CAD build for the part. Positions are in the model's coordinates, mm. A direction names the side the tool comes from. Coordinates: 2 decimals unless noted, no trailing zeros. Write each loop counter-clockwise with the first axis right and the second up, starting at its lowest first coordinate (ties: lowest second). Pieces come first, ordered by that corner, then holes. Notation, with made-up numbers: M 24,-23.5 L 37,-23.5 A35 cw 37,9.5 Z; hole C -40,-18.75 d1. An arc over 180 degrees is marked long. Answer as CSV lines item,"result". Start each with the question number.
```python
from build123d import *

# Parameters (mm, degrees)
F0_W          = 40.64
F0_H          = 40.64
F1_DEPTH      = 23.876
F2_SIZE2      = 10.16
F2_SIZE       = 16.51
F4_DEPTH      = 5.5372
F4_DEPTH_BACK = 35.052
F6_DEPTH      = 0.508
F7_T4_DEPTH   = 41.0469310155
F7_S5_R       = 17.3367265746
F7_T6_DEPTH   = 25
F7_T10_DEPTH  = 41.0469310155
F7_S11_R      = 17.3367265746
F7_T12_DEPTH  = 25
F7_T16_DEPTH  = 41.0469310155
F7_S17_R      = 17.3367265746
F7_T18_DEPTH  = 25
F7_T23_DEPTH  = 41.0469310155
F7_S24_R      = 17.3367265746
F7_T25_DEPTH  = 25
F7_T30_DEPTH  = 41.0469310155
F7_S31_R      = 17.3367265746
F7_T32_DEPTH  = 25
F7_T37_DEPTH  = 41.0469310155
F7_S39_R      = 17.3367265746
F7_T40_DEPTH  = 25
F7_T44_DEPTH  = 41.0469310155
F7_S46_R      = 17.3367265746
F7_T47_DEPTH  = 25
F7_T51_DEPTH  = 41.0469310155
F7_S53_R      = 17.3367265746
F7_T54_DEPTH  = 25


# Not quite as in the source:
# - a fillet or chamfer that OpenCascade refuses, or shapes differently, is made with other operations: its cross-section is extruded or revolved along the edge and cut away or added


with BuildPart() as f1:
    # F0 (on Top) → F1 (new body)
    with BuildSketch(Plane.XY):
        with Locations((-20.32, 14.8309261845)):
            Rectangle(F0_W, F0_H)
    extrude(amount=F1_DEPTH)

    # F2
    f2_edges = [f1.edges().sort_by_distance(p)[0] for p in [
        (0, 14.830926, 23.876),
        (-20.32, 35.150926, 23.876),
        (-40.64, 14.830926, 23.876),
        (-20.32, -5.489074, 23.876),
    ]]
    chamfer(f2_edges, length=F2_SIZE, length2=F2_SIZE2)

    # F3 (on Front) → F4 (join, two sides)
    with BuildSketch(Plane.XZ) as f4_sk:
        with BuildLine():
            Line((-19.622727835, 21.5899987397), (-21.017272165, 21.5899987397))
            ThreePointArc((-21.017272165, 21.5899987397), (-32.4394065874, 17.2953936781), (-38.2026230943, 6.5392734254))
            Line((-38.2026230943, 6.5392734254), (-2.4373769057, 6.5392734254))
            ThreePointArc((-2.4373769057, 6.5392734254), (-8.2005934126, 17.2953936781), (-19.622727835, 21.5899987397))
        make_face()
    extrude(amount=F4_DEPTH)
    extrude(f4_sk.sketch, amount=-F4_DEPTH_BACK)

    # F5 (on face) → F6 (cut)
    with BuildSketch(Plane.XY.offset(23.876)):
        with BuildLine():
            Line((-20.32, 11.3146617191), (-20.32, 20.958676386))
            Line((-20.32, 20.958676386), (-22.098, 20.958676386))
            ThreePointArc((-22.098, 20.958676386), (-22.5080143202, 20.5929218839), (-22.1218966733, 20.2020238648))
            ThreePointArc((-22.1218966733, 20.2020238648), (-20.8577108363, 18.9738562556), (-22.098, 17.7215606446))
            Line((-22.098, 17.7215606446), (-24.7307707736, 12.9957624854))
            ThreePointArc((-24.7307707736, 12.9957624854), (-24.7178678661, 11.8725673854), (-23.7429447999, 11.3146617191))
            Line((-23.7429447999, 11.3146617191), (-20.32, 11.3146617191))
        make_face()
        with BuildLine():
            Line((-18.542, 20.958676386), (-20.32, 20.958676386))
            Line((-20.32, 20.958676386), (-20.32, 11.3146617191))
            Line((-20.32, 11.3146617191), (-16.8970552001, 11.3146617191))
            ThreePointArc((-16.8970552001, 11.3146617191), (-15.9221321339, 11.8725673854), (-15.9092292264, 12.9957624854))
            Line((-15.9092292264, 12.9957624854), (-18.542, 17.7215606446))
            ThreePointArc((-18.542, 17.7215606446), (-19.7822891637, 18.9738562556), (-18.5181033267, 20.2020238648))
            ThreePointArc((-18.5181033267, 20.2020238648), (-18.1319856798, 20.5929218839), (-18.542, 20.958676386))
        make_face()
    extrude(amount=-F6_DEPTH, mode=Mode.SUBTRACT)

    # F7: fillet of radius 5.08 on 4 edges, made by hand


with BuildPart() as f7_tool2:
    # F7_s3 → F7_t4 (new body)
    with BuildSketch(Plane(origin=(-11.8080697784, -11.8080697784, -19.18811339), x_dir=(-0.7071067812, 0.7071067812, 0), z_dir=(0.4642070825, 0.4642070825, 0.7543365091))):
        with BuildLine():
            ThreePointArc((21.7962143454, 27.1330755892), (24.85545827, 28.157532887), (27.9147021947, 27.1330755892))
            Line((27.9147021947, 27.1330755892), (24.85545827, 29.4407749719))
            Line((24.85545827, 29.4407749719), (21.7962143454, 27.1330755892))
        make_face()
    extrude(amount=F7_T4_DEPTH)

    # F7_s5 → F7_t6 (cut, symmetric)
    with BuildSketch(Plane.XZ.offset(-0.8)):
        with Locations((-21.017272165, 4.253272165)):
            Circle(F7_S5_R)
    extrude(amount=F7_T6_DEPTH, both=True, mode=Mode.SUBTRACT)


with BuildPart() as f1_1:
    add(f1.part)

    # F7_t1: cut F7_tool2
    add(f7_tool2.part, mode=Mode.SUBTRACT)


with BuildPart() as f7_tool8:
    # F7_s9 → F7_t10 (new body)
    with BuildSketch(Plane(origin=(3.050628701, -3.050628701, -4.9572716391), x_dir=(-0.7071067812, -0.7071067812, 0), z_dir=(-0.4642070825, 0.4642070825, 0.7543365091))):
        with BuildLine():
            ThreePointArc((0.8221173927, 5.4558434178), (3.8813613174, 6.4803007156), (6.9406052421, 5.4558434178))
            Line((6.9406052421, 5.4558434178), (3.8813613174, 7.7635428005))
            Line((3.8813613174, 7.7635428005), (0.8221173927, 5.4558434178))
        make_face()
    extrude(amount=F7_T10_DEPTH)

    # F7_s11 → F7_t12 (cut, symmetric)
    with BuildSketch(Plane.XZ.offset(-0.8)):
        with Locations((-19.622727835, 4.253272165)):
            Circle(F7_S11_R)
    extrude(amount=F7_T12_DEPTH, both=True, mode=Mode.SUBTRACT)


with BuildPart() as f1_2:
    add(f1_1.part)

    # F7_t7: cut F7_tool8
    add(f7_tool8.part, mode=Mode.SUBTRACT)


with BuildPart() as f7_tool14:
    # F7_s15 → F7_t16 (new body)
    with BuildSketch(Plane(origin=(9.442408336, 9.442408336, -15.3439135461), x_dir=(0.7071067812, -0.7071067812, 0), z_dir=(-0.4642070825, -0.4642070825, 0.7543365091))):
        with BuildLine():
            ThreePointArc((-21.7962143454, 21.2773704954), (-24.85545827, 22.3018277932), (-27.9147021947, 21.2773704954))
            Line((-27.9147021947, 21.2773704954), (-24.85545827, 23.5850698781))
            Line((-24.85545827, 23.5850698781), (-21.7962143454, 21.2773704954))
        make_face()
    extrude(amount=F7_T16_DEPTH)

    # F7_s17 → F7_t18 (cut, symmetric)
    with BuildSketch(Plane.XZ.offset(-28.8)):
        with Locations((-19.622727835, 4.253272165)):
            Circle(F7_S17_R)
    extrude(amount=F7_T18_DEPTH, both=True, mode=Mode.SUBTRACT)

    split(bisect_by=Plane.XZ.offset(-35.052), keep=Keep.BOTTOM)


with BuildPart() as f1_3:
    add(f1_2.part)

    # F7_t13: cut F7_tool14
    add(f7_tool14.part, mode=Mode.SUBTRACT)


with BuildPart() as f7_tool21:
    # F7_s22 → F7_t23 (new body)
    with BuildSketch(Plane(origin=(9.442408336, 9.442408336, -15.3439135461), x_dir=(0.7071067812, -0.7071067812, 0), z_dir=(-0.4642070825, -0.4642070825, 0.7543365091))):
        with BuildLine():
            ThreePointArc((-21.7962143454, 21.2773704954), (-24.85545827, 22.3018277932), (-27.9147021947, 21.2773704954))
            Line((-27.9147021947, 21.2773704954), (-24.85545827, 23.5850698781))
            Line((-24.85545827, 23.5850698781), (-21.7962143454, 21.2773704954))
        make_face()
    extrude(amount=F7_T23_DEPTH)

    # F7_s24 → F7_t25 (intersect, symmetric)
    with BuildSketch(Plane.XZ.offset(-28.8)):
        with Locations((-19.622727835, 4.253272165)):
            Circle(F7_S24_R)
    extrude(amount=F7_T25_DEPTH, both=True, mode=Mode.INTERSECT)

    split(bisect_by=Plane.XZ.offset(-35.052), keep=Keep.BOTTOM)


with BuildPart() as f1_4:
    add(f1_3.part)

    # F7_t20: cut F7_tool21
    add(f7_tool21.part, mode=Mode.SUBTRACT)


with BuildPart() as f7_tool28:
    # F7_s29 → F7_t30 (new body)
    with BuildSketch(Plane(origin=(9.442408336, 9.442408336, -15.3439135461), x_dir=(0.7071067812, -0.7071067812, 0), z_dir=(-0.4642070825, -0.4642070825, 0.7543365091))):
        with BuildLine():
            ThreePointArc((-21.7962143454, 21.2773704954), (-24.85545827, 22.3018277932), (-27.9147021947, 21.2773704954))
            Line((-27.9147021947, 21.2773704954), (-24.85545827, 23.5850698781))
            Line((-24.85545827, 23.5850698781), (-21.7962143454, 21.2773704954))
        make_face()
    extrude(amount=F7_T30_DEPTH)

    # F7_s31 → F7_t32 (cut, symmetric)
    with BuildSketch(Plane.XZ.offset(-28.8)):
        with Locations((-19.622727835, 4.253272165)):
            Circle(F7_S31_R)
    extrude(amount=F7_T32_DEPTH, both=True, mode=Mode.SUBTRACT)

    split(bisect_by=Plane.XZ.offset(-35.052), keep=Keep.TOP)


with BuildPart() as f1_5:
    add(f1_4.part)

    # F7_t27: cut F7_tool28
    add(f7_tool28.part, mode=Mode.SUBTRACT)


with BuildPart() as f7_tool35:
    # F7_s36 → F7_t37 (new body)
    with BuildSketch(Plane(origin=(-18.1998494135, 18.1998494135, -29.5747552969), x_dir=(0.7071067812, 0.7071067812, 0), z_dir=(0.4642070825, -0.4642070825, 0.7543365091))):
        with BuildLine():
            ThreePointArc((-0.8221173927, 42.9546026668), (-3.8813613174, 43.9790599646), (-6.9406052421, 42.9546026668))
            Line((-6.9406052421, 42.9546026668), (-3.8813613174, 45.2623020495))
            Line((-3.8813613174, 45.2623020495), (-0.8221173927, 42.9546026668))
        make_face()
    extrude(amount=F7_T37_DEPTH)

    split(bisect_by=Plane.XZ.offset(-35.052), keep=Keep.BOTTOM)

    # F7_s39 → F7_t40 (cut, symmetric)
    with BuildSketch(Plane.XZ.offset(-28.8)):
        with Locations((-21.017272165, 4.253272165)):
            Circle(F7_S39_R)
    extrude(amount=F7_T40_DEPTH, both=True, mode=Mode.SUBTRACT)


with BuildPart() as f1_6:
    add(f1_5.part)

    # F7_t34: cut F7_tool35
    add(f7_tool35.part, mode=Mode.SUBTRACT)


with BuildPart() as f7_tool42:
    # F7_s43 → F7_t44 (new body)
    with BuildSketch(Plane(origin=(-18.1998494135, 18.1998494135, -29.5747552969), x_dir=(0.7071067812, 0.7071067812, 0), z_dir=(0.4642070825, -0.4642070825, 0.7543365091))):
        with BuildLine():
            ThreePointArc((-0.8221173927, 42.9546026668), (-3.8813613174, 43.9790599646), (-6.9406052421, 42.9546026668))
            Line((-6.9406052421, 42.9546026668), (-3.8813613174, 45.2623020495))
            Line((-3.8813613174, 45.2623020495), (-0.8221173927, 42.9546026668))
        make_face()
    extrude(amount=F7_T44_DEPTH)

    split(bisect_by=Plane.XZ.offset(-35.052), keep=Keep.TOP)

    # F7_s46 → F7_t47 (cut, symmetric)
    with BuildSketch(Plane.XZ.offset(-28.8)):
        with Locations((-21.017272165, 4.253272165)):
            Circle(F7_S46_R)
    extrude(amount=F7_T47_DEPTH, both=True, mode=Mode.SUBTRACT)


with BuildPart() as f1_7:
    add(f1_6.part)

    # F7_t41: cut F7_tool42
    add(f7_tool42.part, mode=Mode.SUBTRACT)


with BuildPart() as f7_tool49:
    # F7_s50 → F7_t51 (new body)
    with BuildSketch(Plane(origin=(-18.1998494135, 18.1998494135, -29.5747552969), x_dir=(0.7071067812, 0.7071067812, 0), z_dir=(0.4642070825, -0.4642070825, 0.7543365091))):
        with BuildLine():
            ThreePointArc((-0.8221173927, 42.9546026668), (-3.8813613174, 43.9790599646), (-6.9406052421, 42.9546026668))
            Line((-6.9406052421, 42.9546026668), (-3.8813613174, 45.2623020495))
            Line((-3.8813613174, 45.2623020495), (-0.8221173927, 42.9546026668))
        make_face()
    extrude(amount=F7_T51_DEPTH)

    split(bisect_by=Plane.XZ.offset(-35.052), keep=Keep.BOTTOM)

    # F7_s53 → F7_t54 (intersect, symmetric)
    with BuildSketch(Plane.XZ.offset(-28.8)):
        with Locations((-21.017272165, 4.253272165)):
            Circle(F7_S53_R)
    extrude(amount=F7_T54_DEPTH, both=True, mode=Mode.INTERSECT)


with BuildPart() as f1_8:
    add(f1_7.part)

    # F7_t48: cut F7_tool49
    add(f7_tool49.part, mode=Mode.SUBTRACT)


solid = f1_8.part
```
1) Tool access for faces 4 (the flat face through (-20, -1, 21.59)), 5 (the flat face through (-20, 31, 21.59)), 6 (the flat face through (-20, 15, 23.368)): list every direction of +Z, -Z, +X, -X, +Y, -Y with a clear straight run to the whole face (end or side of a thin tool).
2) Two-plate mould, pull along X, no slides. Class faces 1 (the cylindrical face through (-10.27, -2.18, 18.85)), 2 (the flat face through (-17.21, 15.33, 23.63)), 3 (the flat face through (-21, -5.537, 12)): pulls with the +X half, pulls with the -X half, needs draft (parallel to the pull), parting line crosses it, or undercut.
3) Band-saw the part on A-A, the plane y = 15. List the corners of the cut face in (x, z).
4) Pin check, flat tips, straight feed: P1, Ø8, axis at y = 21, z = 11.5, coming from the +X side; P2, Ø1.5, axis at x = -20, y = 29.5, coming from the +Z side; P3, Ø4.5, axis at x = -12, z = 12, coming from the +Y side. Stop position of each tip, or through.
5) Band-saw the part on B-B, the plane x = -17.5. List the corners of the cut face in (y, z).
6) Probe L1, parallel to Z at x = -12, y = 30; L2, parallel to Y at x = -11, z = 3.5; L3, parallel to Y at x = -18, z = 16.5. List the from-to ranges inside material, lowest first. Write a range as [from, to].
Result sheet:
1,face 4,"+Z, +X, -X, -Y"
1,face 5,"+Z, +X, -X, +Y"
1,face 6,"+Z"
2,face 1,"pulls with the +X half"
2,face 2,"undercut"
2,face 3,"needs draft"
3,outline,"M -40.64,0 L 0,0 L 0,7.37 L -10.16,23.88 L -17.03,23.88 L -17.03,23.37 L -23.61,23.37 L -23.61,23.88 L -30.48,23.88 L -40.64,7.37 Z"
4,P1,"stops at x = -0.08"
4,P2,"stops at z = 21.59"
4,P3,"stops at y = 35.05"
5,outline,"M -5.54,6.54 L -5.49,6.54 L -5.49,0 L 35.15,0 L 35.15,7.37 L 35.05,7.53 L 35.05,21.46 L 26.48,21.46 L 24.99,23.88 L 15.85,23.88 L 15.85,23.37 L 11.31,23.37 L 11.31,23.88 L 4.67,23.88 L 3.18,21.46 L -5.54,21.46 Z"
6,L1,"z = [0, 19.82]"
6,L2,"y = [-5.49, 35.15]"
6,L3,"y = [-5.54, 35.05]"
